For this review, use the dimensioned drawing (mm, ordinates from the lowest corner) and the shaded views. A direction names the side the tool comes from. Coordinates: 2 decimals unless noted, no trailing zeros. Write each loop counter-clockwise with the first axis right and the second up, starting at its lowest first coordinate (ties: lowest second). Pieces come first, ordered by that corner, then holes.
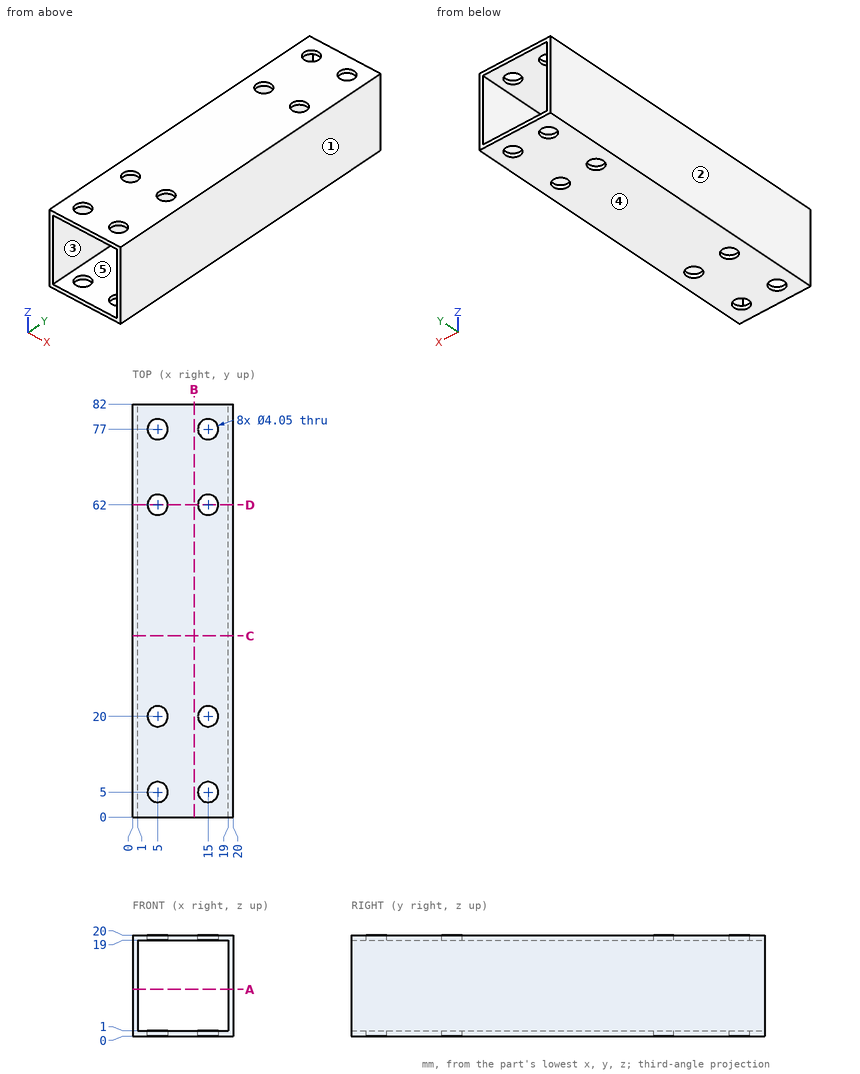
Item 1: Take a section at B-B, the plane x = 12.25. Write out the cut boundary in (y, z).
Solved:
outline: (0, 0) - (82, 0) - (82, 1) - (0, 1) - close; (0, 19) - (82, 19) - (82, 20) - (0, 20) - close
Item 2: To check wall thickness, follow line 1 along Y through (x, z) = (5, 19.7) (3 decimals); line 2 along Z through (x, y) = (5, 52). State the ranges of each line that lie inside material, in increasing order.
Solved:
line 1: y = 0 to 2.975, 7.025 to 17.975, 22.025 to 59.975, 64.025 to 74.975, 79.025 to 82
line 2: z = 0 to 1, 19 to 20
Item 3: Take a section at A-A, the plane z = 9.25. Write out the cut boundary in (x, y).
Solved:
outline: (0, 0) - (1, 0) - (1, 82) - (0, 82) - close; (19, 0) - (20, 0) - (20, 82) - (19, 82) - close
Item 4: Machinability: for the marked faces 4 and 5, which of the approach directions +Z, -Z, +X, -X, +Y, -Y give a long, thin tool a straight path to every point of the face, cutting with its end or side? Answer none if there is none.
Solved:
face 4: -Z, +X, -X, +Y, -Y
face 5: +Y, -Y
Item 5: For pin 1 (2.5 mm diameter, centred on x = 5, y = 62, fed in from -Z), flat-tipped, find the tip position at first contact; note if it passes through.
Solved:
pin 1: passes through
Item 6: Take a section at C-C, the plane y = 36. Write out the cut boundary in (x, z).
Solved:
outline: (0, 0) - (20, 0) - (20, 20) - (0, 20) - close; hole (1, 1) - (19, 1) - (19, 19) - (1, 19) - close
Item 7: Mouldability with a two-part tool opening along X and no side actions: class the marked faces 1, 2 and 3 as pulls with the +X half, pulls with the -X half, needs draft (parallel to the pull), parting line crosses it, or undercut.
Solved:
face 1: pulls with the +X half
face 2: pulls with the -X half
face 3: undercut
Item 8: Take a section at D-D, the plane y = 62. Write out the cut boundary in (x, z) (3 decimals), plus the area to 3 significant figures.
Solved:
outline: (0, 0) - (2.975, 0) - (2.975, 1) - (1, 1) - (1, 19) - (2.975, 19) - (2.975, 20) - (0, 20) - close; (7.025, 0) - (12.975, 0) - (12.975, 1) - (7.025, 1) - close; (7.025, 19) - (12.975, 19) - (12.975, 20) - (7.025, 20) - close; (17.025, 0) - (20, 0) - (20, 20) - (17.025, 20) - (17.025, 19) - (19, 19) - (19, 1) - (17.025, 1) - close
area: 59.8 mm2
